Autodesk Inventor part; units mm, degrees
ref_plane "YZ Plane" through (0, 0, 0) normal (1, 0, 0) x (0, 1, 0)
ref_plane "XZ Plane" through (0, 0, 0) normal (0, 1, 0) x (-1, 0, 0)
ref_plane "XY Plane" through (0, 0, 0) normal (0, 0, 1) x (1, 0, 0)
sketch "Sketch1" plane through (0, 0, 0) normal (0, 1, 0) x (-1, 0, 0)
  circle A0 centre (0, 0) radius 4.2386
  circle A1 centre (0, 0) radius 14.0056
  line L0 (0, 0) -> (0, 22.8956)
  line L1 (0, 0) -> (0, -22.8956)
  line L2 (0, 22.8956) -> (38.1, 22.8956)
  line L3 (0, -22.8956) -> (-38.1, -22.8956)
  line L4 (38.1, 22.8956) -> (-38.1, 22.8956)
  line L5 (-38.1, 22.8956) -> (-38.1, -22.8956)
  line L6 (-38.1, -22.8956) -> (38.1, -22.8956)
  line L7 (38.1, -22.8956) -> (38.1, 22.8956)
  line L8 (19.05, 22.8956) -> (38.1, 22.8956)
  line L9 (38.1, 22.8956) -> (19.05, 22.8956)
  line L10 (19.05, -22.8956) -> (38.1, -22.8956)
  line L11 (38.1, -22.8956) -> (38.1, 22.8956)
  line L12 (38.1, 22.8956) -> (19.05, 22.8956)
  line L13 (19.05, 22.8956) -> (19.05, -22.8956)
  line L14 (38.1, 22.8956) -> (28.575, 22.8956)
  circle A2 centre (28.575, 11.4465) radius 4.445
  circle A3 centre (28.575, -11.4516) radius 4.445
  line L15 (-19.05, -22.8956) -> (-19.05, 22.8956)
  line L16 (-38.1, 22.8956) -> (-19.05, 22.8956)
  line L17 (-19.05, 22.8956) -> (-38.1, 22.8956)
  line L18 (-38.1, -22.8956) -> (-19.05, -22.8956)
  line L19 (-19.05, -22.8956) -> (-19.05, 22.8956)
  line L20 (-19.05, 22.8956) -> (-38.1, 22.8956)
  line L21 (-38.1, 22.8956) -> (-38.1, -22.8956)
  line L22 (-19.05, 22.8956) -> (-28.575, 22.8956)
  circle A4 centre (-28.575, 11.4465) radius 4.445
  circle A5 centre (-28.575, -11.4516) radius 4.445
  dimension "d0" = 8.4772
  dimension "d1" = 28.0111
  dimension "d11" = 22.8956
  dimension "d12" = 22.8956
  dimension "d13" = 38.1
  dimension "d14" = 38.1
  dimension "d15" = 45.7911
  dimension "d16" = 76.2
  dimension "d27" = 45.7911
  dimension "d28" = 19.05
  dimension "d29" = 19.05
  dimension "d30" = 9.525
  dimension "d31" = 8.89
  dimension "d32" = 45.7911
  dimension "d33" = 45.7911
  dimension "d34" = 19.05
  dimension "d35" = 19.05
  dimension "d36" = 9.525
  dimension "d37" = 8.89
sketch "Sketch2" plane through (0, 0, 0) normal (0, 1, 0) x (-1, 0, 0)
  circle A0 centre (0, 0) radius 4.2386
  circle A1 centre (0, 0) radius 14.0056
  line L0 (0, 0) -> (0, 22.8956)
  line L1 (0, 0) -> (0, -22.8956)
  line L2 (0, 22.8956) -> (38.1, 22.8956)
  line L3 (0, -22.8956) -> (-38.1, -22.8956)
  line L4 (38.1, 22.8956) -> (-38.1, 22.8956)
  line L5 (-38.1, 22.8956) -> (-38.1, -22.8956)
  line L6 (-38.1, -22.8956) -> (38.1, -22.8956)
  line L7 (38.1, -22.8956) -> (38.1, 22.8956)
  dimension "d17" = 8.4772
  dimension "d18" = 28.0111
  dimension "d19" = 22.8956
  dimension "d20" = 22.8956
  dimension "d21" = 38.1
  dimension "d22" = 38.1
  dimension "d23" = 45.7911
  dimension "d24" = 76.2
extrude "Extrusion2" add sketch "Sketch2" along normal blind 3.302 contours A0 L0 A1 L1 | A0 L1 A1 L0
extrude "Extrusion3" add sketch "Sketch1" along normal blind 9.652 contours L0 L2 L13 L6 L1 A1 | A1 L1 L3 L15 L4 L0 | L2 L7 L6 L13 | L15 L3 L5 L4
properties part number "bracket for drone"
Model file for the job. Use its own axes, mm. A direction names the side the tool comes from. Coordinates: 2 decimals unless noted, no trailing zeros. Write each loop counter-clockwise with the first axis right and the second up, starting at its lowest first coordinate (ties: lowest second). Pieces come first, ordered by that corner, then holes. Notation, with made-up numbers: (65, 72.25) - (114, 72.25) arc R25 ccw to (114, 107.25) - close; hole circle Ø9 at (25.5, 89). An arc over 180 degrees is marked (long way). Use a Markdown table: item, result. Add a question column.
Item 1: Drop a flat-ended pin along its axis: pin 1 (1.5 mm diameter, centred on x = -7, z = -3.5, fed in from +Y). Give the stop position or say it passes through.
Item 2: Band-saw the part on B-B, the plane z = 0. Write the cut outline in (x, y).
Item 3: Band-saw the part on C-C, the plane y = 2.5. Write the cut outline in (x, z) (1 decimal), and give its area (3 significant figures).
Item 4: 3-axis set-ups, long thin cutter, end or side, ignore diameter. For faces 1 (the face through (-13.359, 6.433, -4.207)), 2 (the face through (-24.134, 4.758, -11.647)): which of +Z, -Z, +X, -X, +Y, -Y reach the whole face in a straight line?
Item 5: Band-saw the part on A-A, the plane x = 0. Write the cut outline in (y, z).
Item 6: Drill centre lines: line 1 along X through (y, z) = (5.25, 0); line 2 along X through (y, z) = (1.5, -10); line 3 along X through (y, z) = (0.75, 12). Where is each one in solid material? Low to high.
Item 7: Band-saw the part on D-D, the plane z = 13. Write the cut outline in (x, y).
Item 8: Two-plate mould, pull along X, no slides. Class faces 3 (the face through (38.1, 5, 0)), 4 (the face through (-24.134, 4.758, 11.251)), 5 (the face through (-38.1, 5, 0)), 6 (the face through (1, 0, 5)): pulls with the +X half, pulls with the -X half, needs draft (parallel to the pull), parting line crosses it, or undercut.
A:
| question | item | result |
|---|---|---|
| 1 | pin 1 | stops at y = 3.3 |
| 2 | outline | (-38.1, 0) - (-4.24, 0) - (-4.24, 3.3) - (-14.01, 3.3) - (-14.01, 9.65) - (-38.1, 9.65) - close; (4.24, 0) - (38.1, 0) - (38.1, 9.65) - (14.01, 9.65) - (14.01, 3.3) - (4.24, 3.3) - close |
| 3 | outline | (-38.1, -22.9) - (38.1, -22.9) - (38.1, 22.9) - (-38.1, 22.9) - close; hole circle Ø8.9 at (-28.6, -11.5); hole circle Ø8.9 at (-28.6, 11.4); hole circle Ø8.5 at (0, 0); hole circle Ø8.9 at (28.6, -11.5); hole circle Ø8.9 at (28.6, 11.4) |
| 3 | area | 3,180 mm² |
| 4 | face 1 | +Y |
| 4 | face 2 | +Y, -Y |
| 5 | outline | (0, -22.9) - (9.65, -22.9) - (9.65, -14.01) - (3.3, -14.01) - (3.3, -4.24) - (0, -4.24) - close; (0, 4.24) - (3.3, 4.24) - (3.3, 14.01) - (9.65, 14.01) - (9.65, 22.9) - (0, 22.9) - close |
| 6 | line 1 | x = -38.1 to -14.01, 14.01 to 38.1 |
| 6 | line 2 | x = -38.1 to -32.78, -24.37 to 24.37, 32.78 to 38.1 |
| 6 | line 3 | x = -38.1 to -32.99, -24.16 to 24.16, 32.99 to 38.1 |
| 7 | outline | (-38.1, 0) - (-32.74, 0) - (-32.74, 9.65) - (-38.1, 9.65) - close; (-24.41, 0) - (24.41, 0) - (24.41, 9.65) - (5.21, 9.65) - (5.21, 3.3) - (-5.21, 3.3) - (-5.21, 9.65) - (-24.41, 9.65) - close; (32.74, 0) - (38.1, 0) - (38.1, 9.65) - (32.74, 9.65) - close |
| 8 | face 3 | pulls with the +X half |
| 8 | face 4 | undercut |
| 8 | face 5 | pulls with the -X half |
| 8 | face 6 | needs draft |
